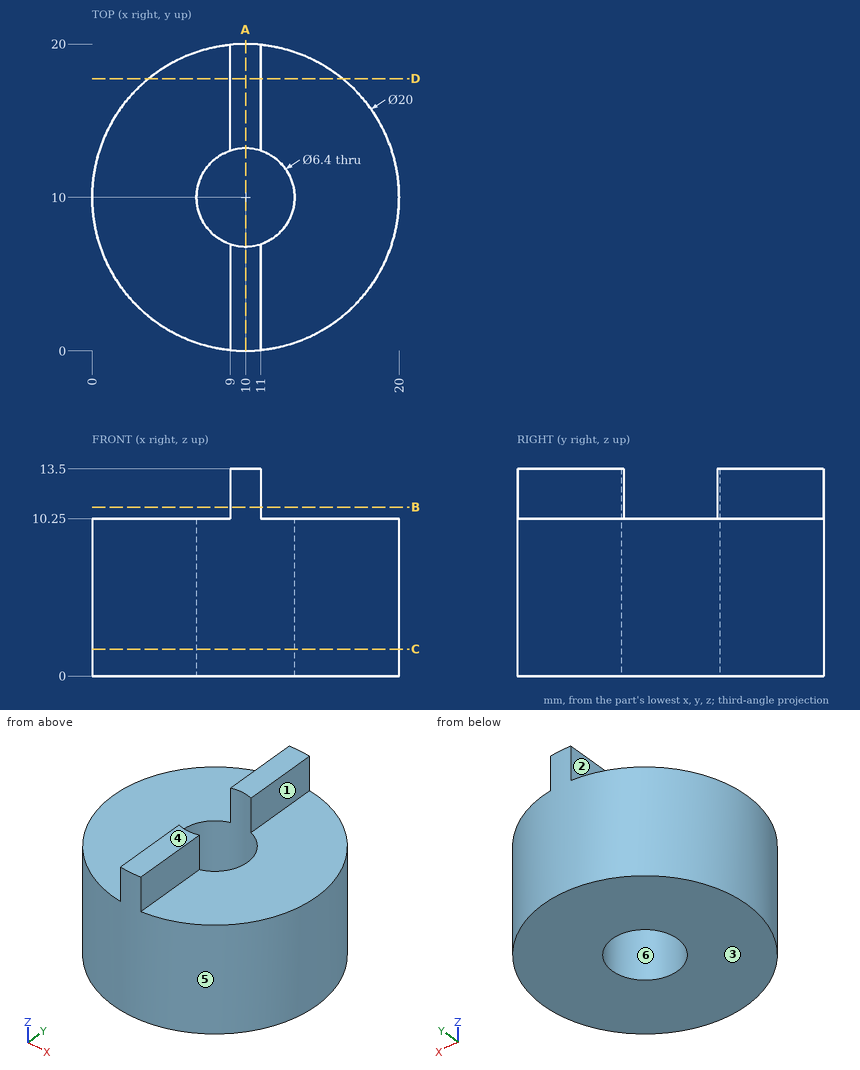
Part print with two shaded views. Sizes in mm from the minimum x, y, z corner. A direction names the side the tool comes from. Coordinates: 2 decimals unless noted, no trailing zeros. Loops run counter-clockwise (first coordinate to the right, second up) from the corner with the lowest first, then second, coordinate; pieces in that order, holes last. Notation, with made-up numbers: M -16.75,79.5 L -4.75,79.5 A26 cw -4.75,112.5 Z; hole C 41,72 d2. An arc over 180 degrees is marked long. Use CSV: the item, a comma, the result in double quotes. Start each with the question number.
1. Band-saw the part on D-D, the plane y = 17.75. List the corners of the cut face in (x, z).
2. Band-saw the part on B-B, the plane z = 11. List the corners of the cut face in (x, y).
3. Flat gauge pins, fed straight in: pin 1 (6 mm diameter, centred on x = 17.5, z = 7, fed in from +Y); pin 2 (3 mm diameter, centred on x = 4.5, y = 17.5, fed in from -Z); pin 3 (4.5 mm diameter, centred on x = 17, y = 5.5, fed in from +Z); pin 4 (1 mm diameter, centred on y = 17, z = 12, fed in from +X). Where does each tip first touch, or does it go through?
4. Band-saw the part on C-C, the plane z = 1.75. List the corners of the cut face in (x, y), then the cut area to 3 significant figures.
5. Probe probe 1 along Y at (x, z) = (10, 5); probe 2 along Z at (x, y) = (17, 7.5). List the from-to ranges inside material, lowest first. Write a range as [from, to].
6. Tool access for the marked faces 1, 2 and 3: list every direction of +Z, -Z, +X, -X, +Y, -Y with a clear straight run to the whole face (end or side of a thin tool).
7. Band-saw the part on A-A, the plane x = 10. List the corners of the cut face in (y, z).
8. Two-plate mould, pull along Y, no slides. Class the marked faces 4, 5 and 6: pulls with the +Y half, pulls with the -Y half, needs draft (parallel to the pull), parting line crosses it, or undercut.
Entries:
1,outline,"M 3.68,0 L 16.32,0 L 16.32,10.25 L 11,10.25 L 11,13.5 L 9,13.5 L 9,10.25 L 3.68,10.25 Z"
2,outline,"M 9,0.05 A10 ccw 11,0.05 L 11,6.96 A3.2 cw 9,6.96 Z; M 9,13.04 A3.2 cw 11,13.04 L 11,19.95 A10 ccw 9,19.95 Z"
3,pin 1,"stops at y = 18.93"
3,pin 2,"stops at z = 0"
3,pin 3,"stops at z = 10.25"
3,pin 4,"stops at x = 11"
4,outline,"C 10,10 d20; hole C 10,10 d6.4"
4,area,"282 mm2"
5,probe 1,"y = [0, 6.8], [13.2, 20]"
5,probe 2,"z = [0, 10.25]"
6,face 1,"+Z, +X, +Y, -Y"
6,face 2,"+Z, -X, +Y, -Y"
6,face 3,"-Z, +X, -X, +Y, -Y"
7,outline,"M 0,0 L 6.8,0 L 6.8,13.5 L 0,13.5 Z; M 13.2,0 L 20,0 L 20,13.5 L 13.2,13.5 Z"
8,face 4,"needs draft"
8,face 5,"parting line crosses it"
8,face 6,"undercut"
